The listing builds one solid part. Answer for the finished solid, in the listing's coordinates (mm). Give positions to 0.01 mm unless a question says otherwise; leave off trailing zeros. Write each loop counter-clockwise with the first axis right and the second up, starting at its lowest first coordinate (ties: lowest second). Pieces come first, ordered by that corner, then holes. Notation, with made-up numbers: (73, 70) - (119, 70) arc R14 ccw to (119, 89) - close; hole circle Ø8 at (58, 66.25). An arc over 180 degrees is marked (long way). Return JSON: item names as keys, results as strings.
from build123d import *

# Parameters (mm, degrees)
SKETCH1_R           = 18.034
BOSS_EXTRUDE1_DEPTH = 2.54
SKETCH2_W           = 2.54
SKETCH2_H           = 2.54
BOSS_EXTRUDE2_DEPTH = 8.89


with BuildPart() as part:
    # Sketch1 → Boss-Extrude1 (new body)
    with BuildSketch(Plane.XY):
        Circle(SKETCH1_R)
    extrude(amount=BOSS_EXTRUDE1_DEPTH)


with BuildPart() as body_2:
    # Sketch2 → Boss-Extrude2 (new body)
    with BuildSketch(Plane(origin=(0, 17.78, 0), x_dir=(1, 0, 0), z_dir=(0, 1, 0))):
        with Locations((0, -1.27)):
            Rectangle(SKETCH2_W, SKETCH2_H)
    extrude(amount=BOSS_EXTRUDE2_DEPTH)


with BuildPart() as part_1:
    add(part.part)

    # Combine1: union body 2
    add(body_2.part)


solid = part_1.part
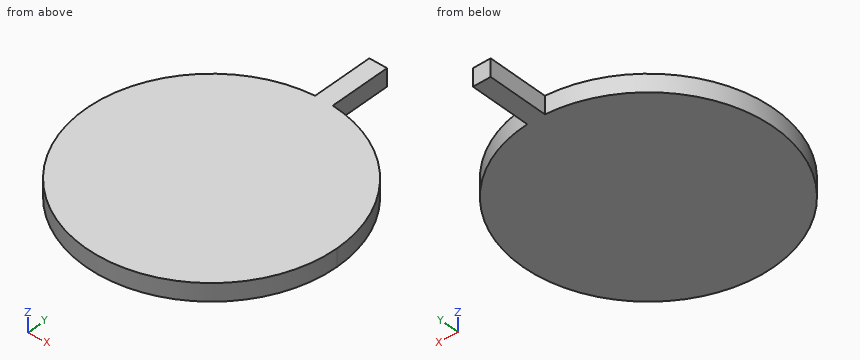
Item 1: Flat-ended cylindrical pins translate along their axes: P1, Ø1, axis at y = 7, z = 0.5, coming from the -X side; P2, Ø1.3, axis at y = 22, z = 2, coming from the +X side; P3, Ø6, axis at x = 13.5, y = -10, coming from the -Z side. Find the tip coordinate at first contact, or state that the pin passes through.
Answer below:
{"P1": "stops at x = -16.82", "P2": "stops at x = 1.27", "P3": "stops at z = 0"}
Item 2: Consider L1, parallel to X at y = 22.5, z = 0.2; L2, parallel to Y at x = 3, z = 0.25; L3, parallel to Y at x = -4, z = 1.5. Determine where each line is inside the solid, lowest interval first.
Answer below:
{"L1": "x = -1.27 to 1.27", "L2": "y = -17.78 to 17.78", "L3": "y = -17.58 to 17.58"}
Item 3: A cutting plane is placed at A-A on z = 0.5. Determine the outline of the cut face in (x, y), then the cut area to 3 significant figures.
Answer below:
{"outline": "(-1.27, 17.99) arc R18.03 ccw (long way) to (1.27, 17.99) - (1.27, 26.67) - (-1.27, 26.67) - close", "area": "1,040 mm²"}
Item 4: A cutting plane is placed at B-B on y = -5.5. Determine the outline of the cut face in (x, z).
Answer below:
{"outline": "(-17.17, 0) - (17.17, 0) - (17.17, 2.54) - (-17.17, 2.54) - close"}
